```python
from build123d import *

# Parameters (mm, degrees)
SKETCH1_W           = 20
SKETCH1_H           = 40
SKETCH1_R           = 2.05
BOSS_EXTRUDE1_DEPTH = 7.9375
CHAMFER1_SIZE       = 2.8


with BuildPart() as part:
    # Sketch1 → Boss-Extrude1 (new body)
    with BuildSketch(Plane(origin=(0, -110.068674648, 0), x_dir=(1, 0, 0), z_dir=(0, 1, 0))):
        with Locations((68.333864278, -62.627324848)):
            Rectangle(SKETCH1_W, SKETCH1_H)
        with Locations(Location((68.333864278, -72.627324848, 0), (0, 0, 270))):
            Circle(SKETCH1_R, mode=Mode.SUBTRACT)
        with Locations(Location((68.333864278, -52.627324848, 0), (0, 0, 270))):
            Circle(SKETCH1_R, mode=Mode.SUBTRACT)
    extrude(amount=BOSS_EXTRUDE1_DEPTH)

    # Chamfer1
    chamfer1_edges = [part.edges().sort_by_distance(p)[0] for p in [
        (68.333864278, -102.131174648, 70.577324848),
        (68.333864278, -102.131174648, 50.577324848),
    ]]
    chamfer(chamfer1_edges, length=CHAMFER1_SIZE)


solid = part.part
```
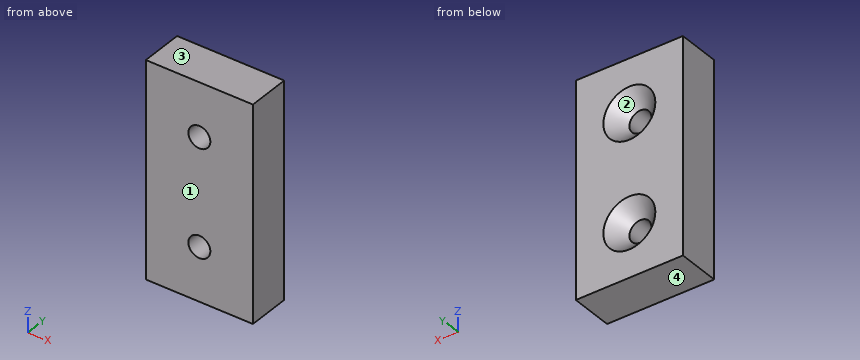
Input: part model. Units: mm. Frame: model coordinates. Face numbers are marked on the shaded views. Coordinates: 2 decimals unless noted, no trailing zeros. Loops run counter-clockwise (first coordinate to the right, second up) from the corner with the lowest first, then second, coordinate; pieces in that order, holes last. Notation, with made-up numbers: (52.25, 5.25) -> (62.25, 5.25) arc R22 cw to (62.25, 39.25) -> close; hole circle Ø3 at (-2.75, 45.25). An arc over 180 degrees is marked (long way). Use a Markdown table: item, result.
1) Material intervals for line 1 along Z through (x, y) = (69.25, -106); line 2 along Z through (x, y) = (64.75, -102.25); line 3 along X through (y, z) = (-109.25, 53), sorted ascending. Write a range as from..to.
Results found:
| item | result |
|---|---|
| line 1 | z = 42.63..50.79, 54.46..70.79, 74.46..82.63 |
| line 2 | z = 42.63..49.54, 55.72..69.54, 75.72..82.63 |
| line 3 | x = 58.33..66.32, 70.35..78.33 |
2) Contact query for flat-ended pins moving along their axis: pin 1 (3.5 mm diameter, centred on x = 68.33, z = 52.63, fed in from -Y); pin 2 (6.5 mm diameter, centred on x = 68.33, z = 72.63, fed in from +Y). Output: stop coordinate, or through.
Results found:
| item | result |
|---|---|
| pin 1 | passes through |
| pin 2 | stops at y = -103.73 |
3) Cut plane C-C (y = -108.25). Return the cut outline in (x, z), then the cut area to 3 significant figures.
Results found:
| item | result |
|---|---|
| outline | (58.33, 42.63) -> (78.33, 42.63) -> (78.33, 82.63) -> (58.33, 82.63) -> close; hole circle Ø4.1 at (68.33, 52.63); hole circle Ø4.1 at (68.33, 72.63) |
| area | 774 mm2 |
4) Cut plane A-A (y = -103.25). Return the cut outline in (x, z).
Results found:
| item | result |
|---|---|
| outline | (58.33, 42.63) -> (78.33, 42.63) -> (78.33, 82.63) -> (58.33, 82.63) -> close; hole circle Ø7.46 at (68.33, 52.63); hole circle Ø7.46 at (68.33, 72.63) |
5) Cut plane B-B (x = 70). Give the number of separate pieces and of enclosed holes in the cut face, then the cut area to 3 significant figures.
Results found:
| item | result |
|---|---|
| separate pieces | 3 |
| enclosed holes | 0 |
| area | 260 mm2 |
6) Pull-direction query (Z, two-part tool) for the marked faces 1, 2, 3 and 4; classes: released by +Z, released by -Z, zero draft, split by the parting line, or undercut.
Results found:
| item | result |
|---|---|
| face 1 | zero draft |
| face 2 | undercut |
| face 3 | released by +Z |
| face 4 | released by -Z |
